Autodesk Inventor part; units mm, degrees
ref_plane "YZ Plane" through (0, 0, 0) normal (1, 0, 0) x (0, 1, 0)
ref_plane "XZ Plane" through (0, 0, 0) normal (0, 1, 0) x (-1, 0, 0)
ref_plane "XY Plane" through (0, 0, 0) normal (0, 0, 1) x (1, 0, 0)
sketch "Boceto1" plane through (0, 0, 0) normal (0, 0, 1) x (1, 0, 0)
  line L0 (0, 0) -> (127.5, 0)
  line L1 (127.5, 0) -> (127.5, 177)
  line L2 (127.5, 177) -> (0, 177)
  line L3 (0, 177) -> (0, 0)
  dimension "d32" = 127.5
  dimension "d33" = 177
extrude "Extrusión1" add sketch "Boceto1" along normal blind 6
ref_plane "Plano de trabajo6" through (0, 88.5, 0) normal (0, -1, 0) x (1, 0, 0)
ref_plane "Plano de trabajo7" through (63.75, 0, 0) normal (-1, 0, 0) x (0, 0, 1)
sketch "Boceto17" plane through (0, 0, 6) normal (0, 0, 1) x (1, 0, 0)
  line L0 (127.5, 0) -> (116, 0)
  line L1 (116, 0) -> (116, 11.5)
  line L2 (116, 11.5) -> (127.5, 11.5)
  line L3 (127.5, 11.5) -> (127.5, 0)
  line L4 (0, 0) -> (11.5, 0)
  line L5 (11.5, 0) -> (11.5, 11.5)
  line L6 (11.5, 11.5) -> (0, 11.5)
  line L7 (0, 11.5) -> (0, 0)
  line L8 (127.5, 177) -> (116, 177)
  line L9 (116, 177) -> (116, 165.5)
  line L10 (116, 165.5) -> (127.5, 165.5)
  line L11 (127.5, 165.5) -> (127.5, 177)
  line L12 (0, 177) -> (11.5, 177)
  line L13 (11.5, 177) -> (11.5, 165.5)
  line L14 (11.5, 165.5) -> (0, 165.5)
  line L15 (0, 165.5) -> (0, 177)
  dimension "d124" = 11.5
  dimension "d125" = 11.5
  dimension "d129" = 11.5
  dimension "d130" = 11.5
  dimension "d131" = 11.5
  dimension "d132" = 11.5
  dimension "d133" = 11.5
  dimension "d134" = 11.5
extrude "Extrusión12" cut sketch "Boceto17" against normal blind 4
sketch "Boceto18" plane through (0, 0, 2) normal (0, 0, 1) x (1, 0, 0)
  line L0 (0, 0) -> (11.5, 0)
  line L1 (11.5, 0) -> (11.5, 11.5)
  line L2 (11.5, 11.5) -> (0, 11.5)
  line L3 (0, 11.5) -> (0, 0)
  line L4 (127.5, 0) -> (116, 0)
  line L5 (116, 0) -> (116, 11.5)
  line L6 (116, 11.5) -> (127.5, 11.5)
  line L7 (127.5, 11.5) -> (127.5, 0)
  line L8 (127.5, 177) -> (116, 177)
  line L9 (116, 177) -> (116, 165.5)
  line L10 (116, 165.5) -> (127.5, 165.5)
  line L11 (127.5, 165.5) -> (127.5, 177)
  line L12 (0, 177) -> (11.5, 177)
  line L13 (11.5, 177) -> (11.5, 165.5)
  line L14 (11.5, 165.5) -> (0, 165.5)
  line L15 (0, 165.5) -> (0, 177)
  line L16 (116, 11.5) -> (127.5, 0)
  line L17 (127.5, 11.5) -> (116, 0)
  circle A0 centre (121.75, 5.75) radius 2
  dimension "d137" = 4
extrude "Extrusión13" cut sketch "Boceto18" against normal blind 3.2 contours A0 L17 L16 | L16 L17 A0 | A0 L16 L17 | L17 L16 A0
mirror "Simetría7" about plane through (63.75, 0, 0) normal (-1, 0, 0) of "Extrusión13"
mirror "Simetría8" about plane through (0, 88.5, 0) normal (0, -1, 0) of "Extrusión13", "Simetría7"
sketch "Boceto19" plane through (0, 0, 6) normal (0, 0, 1) x (1, 0, 0)
  line L0 (0, 0) -> (127.5, 0)
  line L1 (127.5, 0) -> (127.5, 85.5)
  line L2 (127.5, 85.5) -> (0, 85.5)
  line L3 (0, 85.5) -> (0, 0)
  line L4 (127.5, 0) -> (127.5, 177)
  line L5 (0, 85.5) -> (127.5, 85.5)
  line L6 (127.5, 85.5) -> (127.5, 91.5)
  line L7 (127.5, 91.5) -> (0, 91.5)
  line L8 (0, 91.5) -> (0, 85.5)
  line L9 (0, 91.5) -> (127.5, 91.5)
  line L10 (127.5, 91.5) -> (127.5, 177)
  line L11 (127.5, 177) -> (0, 177)
  line L12 (0, 177) -> (0, 91.5)
  dimension "d140" = 127.5
  dimension "d141" = 85.5
  dimension "d142" = 6
extrude "Extrusión14" cut sketch "Boceto19" against normal blind 2.5
sketch "Boceto20" plane through (0, 0, 0) normal (0, 0, -1) x (-1, 0, 0)
  line L0 (-127.5, 165.5) -> (-127.5, 11.5)
  line L1 (-127.5, 88.5) -> (-127.5, 9.25)
  line L2 (-127.5, 0) -> (-127.5, 177)
  line L3 (-127.5, 88.5) -> (-48.25, 88.5) construction
  line L4 (-11.5, 0) -> (-116, 0)
  line L5 (-63.75, 0) -> (-102.75, 0)
  line L6 (-63.75, 0) -> (-24.75, 0) construction
  line L7 (-102.75, 0) -> (-102.75, 9.25)
  line L8 (-127.5, 9.25) -> (-102.75, 9.25)
  line L9 (-102.75, 9.25) -> (-24.75, 9.25)
  line L10 (-24.75, 9.25) -> (-24.75, 167.75)
  line L11 (-24.75, 167.75) -> (-102.75, 167.75)
  line L12 (-102.75, 167.75) -> (-102.75, 9.25)
  line L13 (-102.75, 9.25) -> (-102.75, 25.75)
  line L14 (-102.75, 25.75) -> (-96.25, 25.75)
  circle A0 centre (-96.25, 25.75) radius 2
  point P0 (0, 0)
  point P1 (-127.5, 91.5)
  point P2 (-127.5, 85.5)
  dimension "d145" = 79.25
  dimension "d146" = 90
  dimension "d149" = 39
  dimension "d150" = 180
  dimension "d151" = 78
  dimension "d152" = 158.5
  dimension "d153" = 16.5
  dimension "d154" = 6.5
  dimension "d155" = 4
extrude "Extrusión15" cut sketch "Boceto20" against normal blind 10 contours A0
mirror "Simetría9" about plane through (0, 88.5, 0) normal (0, -1, 0) of "Extrusión15"
mirror "Simetría10" about plane through (63.75, 0, 0) normal (-1, 0, 0) of "Extrusión15", "Simetría9"
sketch "Boceto21" plane through (0, 0, 3.5) normal (0, 0, 1) x (1, 0, 0)
  circle A0 centre (31.25, 25.75) radius 2
  line L0 (31.25, 25.75) -> (24.75, 25.75)
  line L1 (24.75, 25.75) -> (24.75, 32.25)
  line L2 (24.75, 32.25) -> (37.75, 32.25)
  line L3 (37.75, 32.25) -> (37.75, 19.25)
  line L4 (37.75, 19.25) -> (24.75, 19.25)
  line L5 (24.75, 19.25) -> (24.75, 32.25)
  circle A1 centre (96.25, 151.25) radius 2
  line L6 (96.25, 151.25) -> (102.75, 151.25)
  line L7 (96.25, 151.25) -> (102.75, 151.25) construction
  line L8 (102.75, 151.25) -> (102.75, 157.75)
  line L9 (102.75, 157.75) -> (89.75, 157.75)
  line L10 (89.75, 157.75) -> (89.75, 144.75)
  line L11 (89.75, 144.75) -> (102.75, 144.75)
  line L12 (102.75, 144.75) -> (102.75, 157.75)
  line L13 (37.75, 32.25) -> (89.75, 32.25)
  line L14 (89.75, 32.25) -> (89.75, 144.75)
  line L15 (89.75, 144.75) -> (37.75, 144.75)
  line L16 (37.75, 144.75) -> (37.75, 32.25)
  point P0 (0, 0)
  dimension "d158" = 6.5
  dimension "d159" = 6.5
  dimension "d160" = 13
  dimension "d161" = 13
  dimension "d162" = 6.5
  dimension "d163" = 0
  dimension "d164" = 6.5
  dimension "d165" = 90
  dimension "d166" = 13
  dimension "d167" = 13
extrude "Extrusión16" cut sketch "Boceto21" against normal blind 10 contours L16 L15 L14 L13
sketch "Boceto22" plane through (0, 0, 3.5) normal (0, 0, 1) x (1, 0, 0)
  line L0 (0, 165.5) -> (11.5, 165.5)
  line L1 (0, 165.5) -> (11.5, 165.5)
  line L2 (11.5, 165.5) -> (11.5, 177)
  line L3 (11.5, 165.5) -> (11.5, 177)
  line L4 (11.5, 177) -> (116, 177)
  line L5 (116, 177) -> (116, 165.5)
  line L6 (116, 177) -> (116, 165.5)
  line L7 (116, 165.5) -> (127.5, 165.5)
  line L8 (116, 165.5) -> (127.5, 165.5)
  line L9 (127.5, 165.5) -> (127.5, 11.5)
  line L10 (127.5, 165.5) -> (127.5, 11.5)
  line L11 (127.5, 11.5) -> (116, 11.5)
  line L12 (127.5, 11.5) -> (116, 11.5)
  line L13 (116, 11.5) -> (116, 0)
  line L14 (116, 11.5) -> (116, 0)
  line L15 (116, 0) -> (11.5, 0)
  line L16 (11.5, 0) -> (11.5, 11.5)
  line L17 (11.5, 0) -> (11.5, 11.5)
  line L18 (11.5, 11.5) -> (0, 11.5)
  line L19 (11.5, 11.5) -> (0, 11.5)
  line L20 (0, 11.5) -> (0, 165.5)
  line L21 (37.75, 144.75) -> (89.75, 144.75)
  line L22 (89.75, 144.75) -> (89.75, 32.25)
  line L23 (89.75, 32.25) -> (37.75, 32.25)
  line L24 (37.75, 32.25) -> (37.75, 144.75)
  circle A0 centre (31.25, 25.75) radius 2
  line L25 (31.25, 25.75) -> (24.75, 25.75)
  line L26 (24.75, 25.75) -> (24.75, 32.25)
  line L27 (24.75, 32.25) -> (37.75, 32.25)
  line L28 (37.75, 32.25) -> (37.75, 19.25)
  line L29 (37.75, 19.25) -> (24.75, 19.25)
  line L30 (24.75, 19.25) -> (24.75, 32.25)
  circle A1 centre (96.25, 151.25) radius 2
  line L31 (96.25, 151.25) -> (102.75, 151.25)
  line L32 (96.25, 151.25) -> (102.75, 151.25) construction
  line L33 (102.75, 151.25) -> (102.75, 157.75)
  line L34 (102.75, 157.75) -> (89.75, 157.75)
  line L35 (89.75, 157.75) -> (89.75, 144.75)
  line L36 (89.75, 144.75) -> (102.75, 144.75)
  line L37 (102.75, 144.75) -> (102.75, 157.75)
  line L38 (37.75, 32.25) -> (89.75, 32.25)
  line L39 (89.75, 32.25) -> (89.75, 144.75)
  line L40 (89.75, 144.75) -> (37.75, 144.75)
  line L41 (37.75, 144.75) -> (37.75, 32.25)
  line L42 (24.75, 19.25) -> (102.75, 19.25)
  line L43 (102.75, 19.25) -> (102.75, 157.75)
  line L44 (102.75, 157.75) -> (24.75, 157.75)
  line L45 (24.75, 157.75) -> (24.75, 19.25)
  point P0 (0, 0)
  point P1 (0, 0)
  dimension "d170" = 6.5
  dimension "d171" = 6.5
  dimension "d172" = 13
  dimension "d173" = 13
  dimension "d174" = 6.5
  dimension "d175" = 0
  dimension "d176" = 6.5
  dimension "d177" = 90
  dimension "d178" = 13
  dimension "d179" = 13
extrude "Extrusión17" cut sketch "Boceto22" against normal blind 1.5 contours L0 L2 L4 L5 L7 L9 L11 L13 L15 L16 L18 L20
sketch "Boceto23" plane through (0, 0, 2) normal (0, 0, 1) x (1, 0, 0)
  line L0 (0, 0) -> (11.5, 0)
  line L1 (11.5, 0) -> (11.5, 11.5)
  line L2 (11.5, 11.5) -> (0, 11.5)
  line L3 (0, 11.5) -> (0, 0)
  line L4 (127.5, 177) -> (116, 177)
  line L5 (116, 177) -> (116, 165.5)
  line L6 (116, 165.5) -> (127.5, 165.5)
  line L7 (127.5, 165.5) -> (127.5, 177)
  line L8 (11.5, 11.5) -> (116, 11.5)
  line L9 (116, 11.5) -> (116, 165.5)
  line L10 (116, 165.5) -> (11.5, 165.5)
  line L11 (11.5, 165.5) -> (11.5, 11.5)
  line L12 (24.75, 157.75) -> (102.75, 157.75)
  line L13 (102.75, 157.75) -> (102.75, 19.25)
  line L14 (102.75, 19.25) -> (24.75, 19.25)
  line L15 (24.75, 19.25) -> (24.75, 157.75)
  circle A0 centre (31.25, 151.25) radius 2
  line L16 (31.25, 151.25) -> (0, 151.25)
  line L17 (0, 177) -> (0, 0)
  circle A1 centre (96.25, 25.75) radius 2
  line L18 (0, 151.25) -> (11.5, 151.25)
  line L19 (11.5, 151.25) -> (11.5, 25.75)
  line L20 (11.5, 25.75) -> (0, 25.75)
  line L21 (0, 25.75) -> (0, 151.25)
  line L22 (96.25, 25.75) -> (127.5, 25.75)
  line L23 (127.5, 25.75) -> (116, 25.75)
  line L24 (116, 25.75) -> (116, 151.25)
  line L25 (116, 151.25) -> (127.5, 151.25)
  line L26 (127.5, 151.25) -> (127.5, 25.75)
  dimension "d182" = 11.5
  dimension "d183" = 11.5
  dimension "d184" = 11.5
  dimension "d185" = 11.5
extrude "Extrusión18" cut sketch "Boceto23" against normal blind 3 contours L17 L16 L11 L20 | L9 L25 L26 L22
fillet "Empalme1" radius 2 4 edges at (11.5, 151.25, 1) (116, 151.25, 1) (116, 25.75, 1) (11.5, 25.75, 1)
sketch "Boceto24" plane through (0, 0, 3.5) normal (0, 0, 1) x (1, 0, 0)
  line L0 (24.75, 157.75) -> (102.75, 157.75)
  line L1 (102.75, 157.75) -> (102.75, 19.25)
  line L2 (102.75, 19.25) -> (24.75, 19.25)
  line L3 (24.75, 19.25) -> (24.75, 157.75)
  circle A0 centre (31.25, 151.25) radius 2
  circle A1 centre (31.25, 151.25) radius 2
  circle A2 centre (96.25, 151.25) radius 2
  circle A3 centre (96.25, 151.25) radius 2
  circle A4 centre (96.25, 25.75) radius 2
  circle A5 centre (96.25, 25.75) radius 2
  circle A6 centre (31.25, 25.75) radius 2
  circle A7 centre (31.25, 25.75) radius 2
  line L4 (37.75, 144.75) -> (89.75, 144.75)
  line L5 (89.75, 144.75) -> (89.75, 32.25)
  line L6 (89.75, 32.25) -> (37.75, 32.25)
  line L7 (37.75, 32.25) -> (37.75, 144.75)
  point P0 (0, 0)
extrude "Extrusión19" add sketch "Boceto24" along normal blind 3
sketch "Boceto25" plane through (0, 0, 6.5) normal (0, 0, 1) x (1, 0, 0)
  line L0 (37.75, 144.75) -> (24.75, 144.75)
  line L1 (24.75, 144.75) -> (24.75, 157.75)
  line L2 (24.75, 157.75) -> (37.75, 157.75)
  line L3 (37.75, 157.75) -> (37.75, 144.75)
  line L4 (24.75, 19.25) -> (37.75, 19.25)
  line L5 (37.75, 19.25) -> (37.75, 32.25)
  line L6 (37.75, 32.25) -> (24.75, 32.25)
  line L7 (24.75, 32.25) -> (24.75, 19.25)
  line L8 (102.75, 19.25) -> (89.75, 19.25)
  line L9 (89.75, 19.25) -> (89.75, 32.25)
  line L10 (89.75, 32.25) -> (102.75, 32.25)
  line L11 (102.75, 32.25) -> (102.75, 19.25)
  line L12 (102.75, 157.75) -> (89.75, 157.75)
  line L13 (89.75, 157.75) -> (89.75, 144.75)
  line L14 (89.75, 144.75) -> (102.75, 144.75)
  line L15 (102.75, 144.75) -> (102.75, 157.75)
  circle A0 centre (31.25, 151.25) radius 2
  circle A1 centre (31.25, 151.25) radius 2
  circle A2 centre (96.25, 151.25) radius 2
  circle A3 centre (96.25, 151.25) radius 2
  circle A4 centre (96.25, 25.75) radius 2
  circle A5 centre (96.25, 25.75) radius 2
  circle A6 centre (31.25, 25.75) radius 2
  circle A7 centre (31.25, 25.75) radius 2
  point P0 (0, 0)
  dimension "d191" = 13
  dimension "d192" = 13
sketch "Boceto26" plane through (0, 0, 6.5) normal (0, 0, 1) x (1, 0, 0)
  line L0 (37.75, 32.25) -> (45.75, 32.25)
  line L1 (45.75, 32.25) -> (45.75, 40.25)
  line L2 (45.75, 40.25) -> (37.75, 40.25)
  line L3 (37.75, 40.25) -> (37.75, 32.25)
  line L4 (37.75, 40.25) -> (45.75, 32.25)
  line L5 (89.75, 32.25) -> (81.75, 32.25)
  line L6 (81.75, 32.25) -> (81.75, 40.25)
  line L7 (81.75, 40.25) -> (89.75, 40.25)
  line L8 (89.75, 40.25) -> (89.75, 32.25)
  line L9 (89.75, 40.25) -> (81.75, 32.25)
  line L10 (37.75, 144.75) -> (45.75, 144.75)
  line L11 (45.75, 144.75) -> (45.75, 136.75)
  line L12 (45.75, 136.75) -> (37.75, 136.75)
  line L13 (37.75, 136.75) -> (37.75, 144.75)
  line L14 (45.75, 144.75) -> (37.75, 136.75)
  line L15 (89.75, 144.75) -> (81.75, 144.75)
  line L16 (81.75, 144.75) -> (81.75, 136.75)
  line L17 (81.75, 136.75) -> (89.75, 136.75)
  line L18 (89.75, 136.75) -> (89.75, 144.75)
  line L19 (89.75, 136.75) -> (81.75, 144.75)
  point P0 (0, 0)
  dimension "d193" = 8
  dimension "d194" = 8
  dimension "d195" = 8
  dimension "d196" = 8
  dimension "d197" = 8
  dimension "d198" = 8
  dimension "d199" = 8
  dimension "d200" = 8
extrude "Extrusión20" add sketch "Boceto26" against normal blind 6.5 contours L3 L4 L0 | L5 L9 L8 | L10 L14 L13 | L18 L19 L15
extrude "Extrusión21" cut sketch "Boceto25" against normal blind 3
fillet "Empalme2" radius 1 4 edges at (89.75, 32.25, 5) (37.75, 32.25, 5) (37.75, 144.75, 5) (89.75, 144.75, 5)
properties part number "transillum_diffusor_partE_v1"
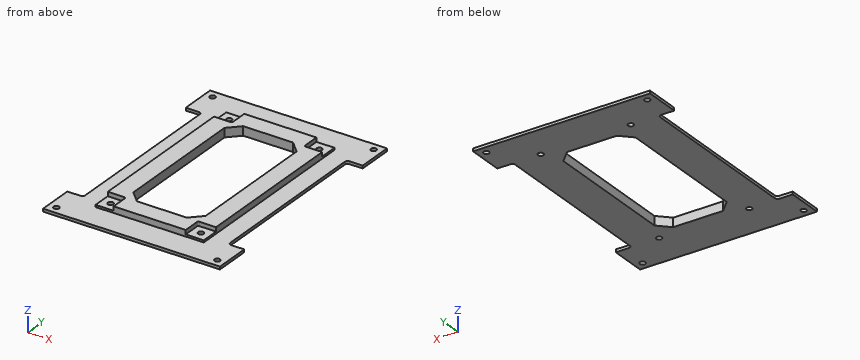
Input: part model. Units: mm. Frame: model coordinates. Give positions to 0.01 mm unless a question says otherwise; leave off trailing zeros. Order: outer loops, then holes, each group sorted by start corner. A loop starts at its lowest first (then second) coordinate and runs counter-clockwise, first axis right, second up.
Q1. Section C-C on y = 110. Output: boundary loops of the cut face in (x, z), and give its area (3 significant figures).
Checked values:
outline: (11.5, 0) - (37.75, 0) - (37.75, 6.5) - (24.75, 6.5) - (24.75, 2) - (11.5, 2) - close; (89.75, 0) - (116, 0) - (116, 2) - (102.75, 2) - (102.75, 6.5) - (89.75, 6.5) - close
area: 222 mm2
Q2. Section B-B on y = 171.25. Output: boundary loops of the cut face in (x, z), and give its area (3 significant figures).
Checked values:
outline: (0, 0) - (3.75, 0) - (3.75, 2) - (0, 2) - close; (7.75, 0) - (119.75, 0) - (119.75, 2) - (7.75, 2) - close; (123.75, 0) - (127.5, 0) - (127.5, 2) - (123.75, 2) - close
area: 239 mm2
Q3. Ray query, probe 1 along Y at (x, z) = (31.25, 1.6); probe 2 along X at (y, z) = (5.75, 1.55); probe 3 along Y at (x, z) = (5.75, 0.6). Return the intervals inside material, ascending.
Checked values:
probe 1: y = 0 to 23.75, 27.75 to 149.25, 153.25 to 177
probe 2: x = 0 to 3.75, 7.75 to 119.75, 123.75 to 127.5
probe 3: y = 0 to 3.75, 7.75 to 25.75, 151.25 to 169.25, 173.25 to 177
Q4. Section D-D on z = 5.25. Output: boundary loops of the cut face in (x, y).
Checked values:
outline: (24.75, 32.25) - (36.75, 32.25) arc R1 cw to (37.75, 31.25) - (37.75, 19.25) - (89.75, 19.25) - (89.75, 31.25) arc R1 cw to (90.75, 32.25) - (102.75, 32.25) - (102.75, 144.75) - (90.75, 144.75) arc R1 cw to (89.75, 145.75) - (89.75, 157.75) - (37.75, 157.75) - (37.75, 145.75) arc R1 cw to (36.75, 144.75) - (24.75, 144.75) - close; hole (37.75, 40.25) - (45.75, 32.25) - (81.75, 32.25) - (89.75, 40.25) - (89.75, 136.75) - (81.75, 144.75) - (45.75, 144.75) - (37.75, 136.75) - close
Q5. Section A-A on x = 40. Output: boundary loops of the cut face in (y, z), and give its area (3 significant figures).
Checked values:
outline: (0, 0) - (38, 0) - (38, 6.5) - (19.25, 6.5) - (19.25, 2) - (0, 2) - close; (139, 0) - (177, 0) - (177, 2) - (157.75, 2) - (157.75, 6.5) - (139, 6.5) - close
area: 321 mm2
Q6. Contact query for flat-ended pins moving along their axis: pin 1 Ø2.5 at (y, z) = (152, 5) entering from -X; pin 2 Ø0.9 at (y, z) = (150, 5.5) entering from +X; pin 3 Ø3 at (y, z) = (94, 1) entering from -X; pin 4 Ø4 at (x, y) = (108, 69) entering from -Z. Output: stop coordinate, or through.
Checked values:
pin 1: stops at x = 37.75
pin 2: stops at x = 89.75
pin 3: stops at x = 11.5
pin 4: stops at z = 0
